Verification items for the finished model (mm, model axes). Face numbers are marked on the shaded views. A direction names the side the tool comes from. Coordinates: 2 decimals unless noted, no trailing zeros. Loops run counter-clockwise (first coordinate to the right, second up) from the corner with the lowest first, then second, coordinate; pieces in that order, holes last. Notation, with made-up numbers: (42, 19) - (61, 19) arc R18 ccw to (61, 36) - close; hole circle Ø3 at (-22.5, 5). An arc over 180 degrees is marked (long way). Answer as CSV lines item,"result". Start each with the question number.
1. Cross-section at C-C (y = 0). Enter the section's corners in (x, z).
2. Gauge pin test, flat ends, axial feed: P1, Ø6, axis at x = -1.5, z = 30, coming from the -Y side; P2, Ø2.5, axis at x = 15.5, y = 0, coming from the +Z side; P3, Ø6, axis at x = -15, y = -8.5, coming from the +Z side. Record the tip position at first contact, or that the pin passes through.
3. Material ranges on line 1 (Y direction, x = -12, z = 32); line 2 (Z direction, x = -0.5, y = 10.25); line 3 (Z direction, x = 2, y = -1), recorded low to high. Write a range as [from, to].
4. Cross-section at A-A (z = 30). Enter the section's corners in (x, y).
5. Cross-section at D-D (x = -12). Enter the section's corners in (y, z).
6. Cross-section at B-B (x = 16). Enter the section's corners in (y, z).
7. Set-up check for the marked faces 1 and 2: record each of +Z, -Z, +X, -X, +Y, -Y from which the full face is reachable in a straight line by a thin tool's end or side.
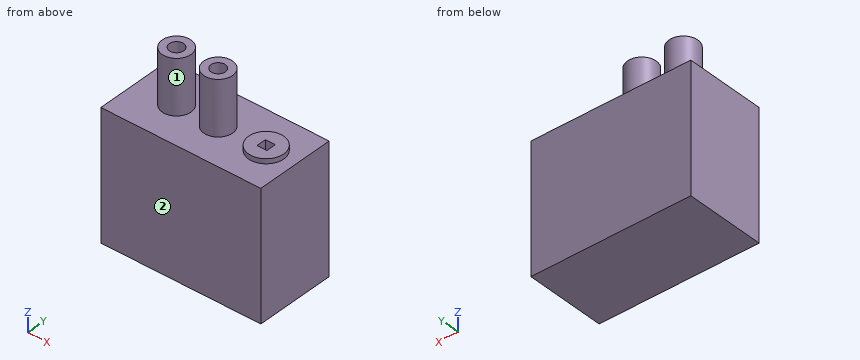
```python
from build123d import *

# Parameters (mm, degrees)
F0_W     = 50
F0_H     = 25
F1_DEPTH = 20
F2_R     = 5.5
F3_DEPTH = 1.5
F2_R_2   = 4.5
F4_DEPTH = 17
F5_W     = 3.1
F5_H     = 3.1
F6_DEPTH = 7.3
F7_R     = 2.25
F8_DEPTH = 17.4


with BuildPart() as f1:
    # F0 (on Top) → F1 (new body, symmetric)
    with BuildSketch(Plane.XY):
        Rectangle(F0_W, F0_H)
    extrude(amount=F1_DEPTH, both=True)

    # F2 (on face) → F3 (join)
    with BuildSketch(Plane.XY.offset(20)):
        with Locations((16, 0)):
            Circle(F2_R)
    extrude(amount=F3_DEPTH)

    # F2 (on face) → F4 (join)
    with BuildSketch(Plane.XY.offset(20)):
        with Locations((-12, 0)):
            Circle(F2_R_2)
        with Locations((1, 0)):
            Circle(F2_R_2)
    extrude(amount=F4_DEPTH)

    # F5 (on face) → F6 (cut)
    with BuildSketch(Plane.XY.offset(21.5)):
        with Locations((16, 0)):
            Rectangle(F5_W, F5_H)
    extrude(amount=-F6_DEPTH, mode=Mode.SUBTRACT)

    # F7 (on face) → F8 (cut)
    with BuildSketch(Plane.XY.offset(37)):
        with Locations((-12, 0)):
            Circle(F7_R)
        with Locations((1, 0)):
            Circle(F7_R)
    extrude(amount=-F8_DEPTH, mode=Mode.SUBTRACT)


solid = f1.part
```
Values follow:
1,outline,"(-25, -20) - (25, -20) - (25, 20) - (21.5, 20) - (21.5, 21.5) - (17.55, 21.5) - (17.55, 14.2) - (14.45, 14.2) - (14.45, 21.5) - (10.5, 21.5) - (10.5, 20) - (5.5, 20) - (5.5, 37) - (3.25, 37) - (3.25, 19.6) - (-1.25, 19.6) - (-1.25, 37) - (-3.5, 37) - (-3.5, 20) - (-7.5, 20) - (-7.5, 37) - (-9.75, 37) - (-9.75, 19.6) - (-14.25, 19.6) - (-14.25, 37) - (-16.5, 37) - (-16.5, 20) - (-25, 20) - close"
2,P1,"stops at y = -4.5"
2,P2,"stops at z = 21.5"
2,P3,"stops at z = 20"
3,line 1,"y = [-4.5, -2.25], [2.25, 4.5]"
3,line 2,"z = [-20, 20]"
3,line 3,"z = [-20, 19.6]"
4,outline,"circle Ø9 at (-12, 0); circle Ø9 at (1, 0); hole circle Ø4.5 at (-12, 0); hole circle Ø4.5 at (1, 0)"
5,outline,"(-12.5, -20) - (12.5, -20) - (12.5, 20) - (4.5, 20) - (4.5, 37) - (2.25, 37) - (2.25, 19.6) - (-2.25, 19.6) - (-2.25, 37) - (-4.5, 37) - (-4.5, 20) - (-12.5, 20) - close"
6,outline,"(-12.5, -20) - (12.5, -20) - (12.5, 20) - (5.5, 20) - (5.5, 21.5) - (1.55, 21.5) - (1.55, 14.2) - (-1.55, 14.2) - (-1.55, 21.5) - (-5.5, 21.5) - (-5.5, 20) - (-12.5, 20) - close"
7,face 1,"+Z"
7,face 2,"+Z, -Z, +X, -X, -Y"
